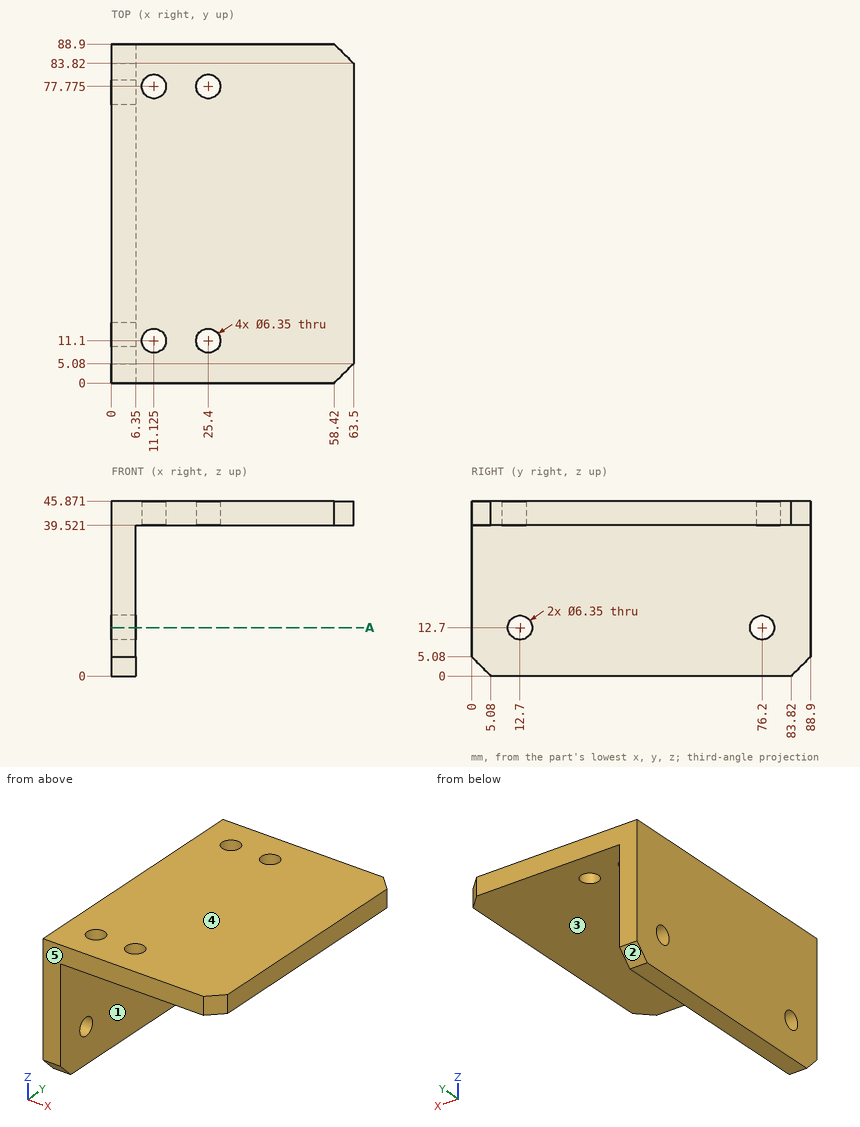
Job drawing, mm, ordinate dimensions from the low corner. One solid piece. A direction names the side the tool comes from. Coordinates: 2 decimals unless noted, no trailing zeros. Answer in a Markdown table with one row per item. Add a question column.
Q1. Wall check: line 1 along Y through (x, z) = (11, 44); line 2 along Z through (x, y) = (2.25, 12.7) (1 decimal); line 3 along Z through (x, y) = (11, 53). Give the ranges that are in metal, low to high. Write a range as [from, to].
Q2. Mould opens along Z. For the marked faces 3, 4 and 5 say: +Z half, -Z half, draft (parallel to the pull), parting line (faces both ways), or undercut.
Q3. Band-saw the part on A-A, the plane z = 12.7. Give the number of separate pieces and of enclosed holes in the cut face, then the cut area to 3 significant figures.
Q4. Which spindle directions (+Z, -Z, +X, -X, +Y, -Y) get a long thin tool onto all of the face, cutting with end or side? Do the marked faces 1 and 2. Say none if no direction does.
Q5. Drop flat-ended pins along their axis: pin 1 (3 mm diameter, centred on y = 35, z = 5, fed in from +X); pin 2 (8 mm diameter, centred on x = 33.5, y = 58.5, fed in from -Z). Give the stop position or say it passes through.
Answers follow:
| question | item | result |
|---|---|---|
| 1 | line 1 | [0, 7.93], [14.27, 74.6], [80.95, 88.9] |
| 1 | line 2 | [0, 9.5], [15.9, 45.9] |
| 1 | line 3 | [39.52, 45.87] |
| 2 | face 3 | -Z half |
| 2 | face 4 | +Z half |
| 2 | face 5 | draft |
| 3 | separate pieces | 3 |
| 3 | enclosed holes | 0 |
| 3 | area | 484 mm^2 |
| 4 | face 1 | -Z, +X, +Y, -Y |
| 4 | face 2 | -Z, +X, -X, +Y |
| 5 | pin 1 | x = 6.35 |
| 5 | pin 2 | z = 39.52 |
